from build123d import *

# Parameters (mm, degrees)
BOSS_EXTRUDE1_DEPTH = 46
SKETCH3_W           = 23
SKETCH3_H           = 15
CUT_EXTRUDE2_DEPTH  = 28
SKETCH4_W           = 23
SKETCH4_H           = 13.957917361
CUT_EXTRUDE3_DEPTH  = 69
SKETCH8_W           = 15.108089283
SKETCH8_H           = 2.529188453
CUT_EXTRUDE4_DEPTH  = 5
SKETCH9_R           = 2.111646756
CUT_EXTRUDE5_DEPTH  = 22
SKETCH7_R           = 11
SKETCH7_R_2         = 4.5
BOSS_EXTRUDE2_DEPTH = 5
BOSS_EXTRUDE3_DEPTH = 5


with BuildPart() as part:
    # Sketch1 → Boss-Extrude1 (new body)
    with BuildSketch(Plane.XY):
        with BuildLine():
            Line((-22.718454064, 23.966100395), (13.281542119, 23.93479699))
            Line((13.281542119, 23.93479699), (13.281542119, -13.210798183))
            Line((13.281542119, -13.210798183), (5.281545459, -13.210798183))
            Line((5.281545459, -13.210798183), (5.281545459, -14.529188453))
            Line((5.281545459, -14.529188453), (-9.718454064, -14.529188453))
            ThreePointArc((-9.718454064, -14.529188453), (-14.925713646, -13.200176165), (-19.056981743, -9.762960731))
            ThreePointArc((-19.056981743, -9.762960731), (-21.779979177, -4.437922335), (-22.718454064, 1.468854607))
            Line((-22.718454064, 1.468854607), (-22.718454064, 23.966100395))
        make_face()
        with BuildLine():
            Line((-18.718455971, 7.468114556), (0.281544029, 7.468114556))
            Line((0.281544029, 7.468114556), (0.281544029, -11.529558479))
            Line((0.281544029, -11.529558479), (-9.718454064, -11.529558479))
            ThreePointArc((-9.718454064, -11.529558479), (-13.398330557, -10.623193541), (-16.168405236, -8.036752998))
            ThreePointArc((-16.168405236, -8.036752998), (-18.168441603, -3.478446477), (-18.718455971, 1.468854607))
            Line((-18.718455971, 1.468854607), (-18.718455971, 7.468114556))
        make_face(mode=Mode.SUBTRACT)
    extrude(amount=BOSS_EXTRUDE1_DEPTH)

    # Sketch3 → Cut-Extrude2 (cut)
    with BuildSketch(Plane.XZ.offset(14.529188453)):
        with Locations((-11.218454064, 31.5)):
            Rectangle(SKETCH3_W, SKETCH3_H)
    extrude(amount=-CUT_EXTRUDE2_DEPTH, mode=Mode.SUBTRACT)

    # Sketch4 → Cut-Extrude3 (cut)
    with BuildSketch(Plane.XZ.offset(14.529188453)):
        with Locations((-11.218454064, 6.978958681)):
            Rectangle(SKETCH4_W, SKETCH4_H)
    extrude(amount=-CUT_EXTRUDE3_DEPTH, mode=Mode.SUBTRACT)

    # Sketch8 → Cut-Extrude4 (cut)
    with BuildSketch(Plane.ZY.offset(22.718454064)):
        with Locations((31.445955359, 14.735405774)):
            Rectangle(SKETCH8_W, SKETCH8_H)
    extrude(amount=-CUT_EXTRUDE4_DEPTH, mode=Mode.SUBTRACT)

    # Sketch9 → Cut-Extrude5 (cut)
    with BuildSketch(Plane.XZ.offset(-13.470811547)):
        with Locations(Location((-9.718454064, 31.5, 0), (0, 0, 270))):
            Circle(SKETCH9_R)
    extrude(amount=-CUT_EXTRUDE5_DEPTH, mode=Mode.SUBTRACT)



with BuildPart() as body_2:
    # Sketch7 → Boss-Extrude2 (new body)
    with BuildSketch(Plane(origin=(0, 16, 0), x_dir=(1, 0, 0), z_dir=(0, 1, 0))):
        with Locations(Location((0.281545936, 17.870886738, 0), (0, 0, 270))):
            Circle(SKETCH7_R)
        with Locations(Location((0.281545936, 17.870886738, 0), (0, 0, 270))):
            Circle(SKETCH7_R_2, mode=Mode.SUBTRACT)
    extrude(amount=-BOSS_EXTRUDE2_DEPTH)


with BuildPart() as part_1:
    add(part.part)

    add(body_2.part)  # Boss-Extrude3 merges body 2
    # Sketch10 → Boss-Extrude3 (add)
    with BuildSketch(Plane(origin=(0, 16, 0), x_dir=(1, 0, 0), z_dir=(0, 1, 0))):
        with BuildLine():
            Line((0.281545936, 0), (0.281545936, 6.870886738))
            ThreePointArc((0.281545936, 6.870886738), (3.700951455, 7.415856087), (6.781544028, 8.996765665))
            Line((6.781544028, 8.996765665), (6.781544028, 0))
            Line((6.781544028, 0), (0.281545936, 0))
        make_face()
    extrude(amount=-BOSS_EXTRUDE3_DEPTH)


solid = part_1.part
CAD build for the part. Positions are in the model's coordinates, mm. A direction names the side the tool comes from. Give positions to 0.01 mm unless a question says otherwise; leave off trailing zeros. Write each loop counter-clockwise with the first axis right and the second up, starting at its lowest first coordinate (ties: lowest second). Pieces come first, ordered by that corner, then holes. Notation, with made-up numbers: (2.25, 54.5) -> (12.25, 54.5) arc R5 cw to (12.25, 61.5) -> close; hole circle Ø2 at (-22.75, -31.75). An arc over 180 degrees is marked (long way). Return JSON: item names as keys, results as strings.
Item 1: Band-saw the part on D-D (z = 18). List the corners of the cut face in (x, y), then the cut area to 3 significant figures.
Answer below:
{"outline": "(-22.72, 1.47) arc R19.06 ccw to (-19.06, -9.76) arc R12.2 ccw to (-9.72, -14.53) -> (5.28, -14.53) -> (5.28, -13.21) -> (13.28, -13.21) -> (13.28, 23.93) -> (-22.72, 23.97) -> close; hole (-18.72, 1.47) arc R16.5 ccw to (-16.17, -8.04) arc R7.52 ccw to (-9.72, -11.53) -> (0.28, -11.53) -> (0.28, 7.47) -> (-18.72, 7.47) -> close", "area": "992 mm2"}
Item 2: Tool access for faces 1 (the cylindrical face through (1.633, 13.535, -13.579)), 2 (the flat face through (-7, 13.471, 32)), 3 (the flat face through (-9, 7.468, 19)): list every direction of +Z, -Z, +X, -X, +Y, -Y with a clear straight run to the whole face (end or side of a thin tool).
Answer below:
{"face 1": "+Y, -Y", "face 2": "-X, -Y", "face 3": "+Z, -Z"}
Item 3: Band-saw the part on B-B (y = 20). List the corners of the cut face in (x, z), then the cut area to 3 significant figures.
Answer below:
{"outline": "(-22.72, 13.96) -> (0.28, 13.96) -> (0.28, 0) -> (13.28, 0) -> (13.28, 46) -> (-22.72, 46) -> close; hole circle Ø4.22 at (-9.72, 31.5)", "area": "1,320 mm2"}
Item 4: Drill centre lines: probe 1 along X at (y, z) = (20, 31.5); probe 2 along X at (y, z) = (2, 23); probe 3 along Y at (x, z) = (-1.5, 15). Where is each one in solid material? Low to high.
Answer below:
{"probe 1": "x = -22.72 to -11.83, -7.61 to 13.28", "probe 2": "x = -22.72 to -18.72, 0.28 to 13.28", "probe 3": "y = -14.53 to -11.53, 7.47 to 23.95"}
Item 5: Band-saw the part on C-C (x = -2). List the corners of the cut face in (y, z).
Answer below:
{"outline": "(-14.53, 13.96) -> (-11.53, 13.96) -> (-11.53, 24) -> (-14.53, 24) -> close; (-14.53, 39) -> (-11.53, 39) -> (-11.53, 46) -> (-14.53, 46) -> close; (7.47, 13.96) -> (23.95, 13.96) -> (23.95, 46) -> (7.47, 46) -> (7.47, 39) -> (13.47, 39) -> (13.47, 24) -> (7.47, 24) -> close; (11, -28.63) -> (16, -28.63) -> (16, -21.75) -> (11, -21.75) -> close; (11, -13.99) -> (16, -13.99) -> (16, -7.11) -> (11, -7.11) -> close"}
Item 6: Drop flat-ended pins along their axis: pin 1 (2 mm diameter, centred on x = -5, z = 42, fed in from +Y); pin 2 (7 mm diameter, centred on x = -14, y = 8, fed in from -Z); pin 3 (17.5 mm diameter, centred on x = -4.5, z = -12.5, fed in from +Y). Give the stop position or say it passes through.
Answer below:
{"pin 1": "stops at y = 23.95", "pin 2": "stops at z = 13.96", "pin 3": "stops at y = 16"}
Item 7: Band-saw the part on A-A (z = 30.5). List the corners of the cut face in (x, y).
Answer below:
{"outline": "(-22.72, 16) -> (-17.72, 16) -> (-17.72, 13.47) -> (-11.58, 13.47) -> (-11.58, 23.96) -> (-22.72, 23.97) -> close; (-7.86, 13.47) -> (0.28, 13.47) -> (0.28, -14.53) -> (5.28, -14.53) -> (5.28, -13.21) -> (13.28, -13.21) -> (13.28, 23.93) -> (-7.86, 23.95) -> close"}
Item 8: Two-plate mould, pull along Y, no slides. Class faces 4 (the flat face through (0, 16, -11)), 5 (the cylindrical face through (-13.35, -10.65, 42.45)), 6 (the flat face through (0.282, 5, 6)): +Y half, -Y half, draft (parallel to the pull), parting line (faces both ways), or undercut.
Answer below:
{"face 4": "+Y half", "face 5": "undercut", "face 6": "draft"}
